For this review, take the finished solid that the model builds, in its own axes (mm). A direction names the side the tool comes from. Give positions to 0.01 mm unless a question says otherwise; leave off trailing zeros. Order: outer loops, then holes, each group sorted by start corner. A loop starts at its lowest first (then second) coordinate and runs counter-clockwise, first axis right, second up.
from build123d import *

# Parameters (mm, degrees)
SKETCH1_W           = 20
SKETCH1_H           = 90
BOSS_EXTRUDE1_DEPTH = 30
SKETCH2_W           = 40
SKETCH2_H           = 40
BOSS_EXTRUDE2_DEPTH = 20
FILLET1_R           = 10


with BuildPart() as part:
    # Sketch1 → Boss-Extrude1 (new body)
    with BuildSketch(Plane.XY):
        with Locations((-20, -45)):
            Rectangle(SKETCH1_W, SKETCH1_H)
    extrude(amount=BOSS_EXTRUDE1_DEPTH)

    # Sketch2 → Boss-Extrude2 (add)
    with BuildSketch(Plane.XY):
        with Locations((-10, -70)):
            Rectangle(SKETCH2_W, SKETCH2_H)
    extrude(amount=-BOSS_EXTRUDE2_DEPTH)

    # Fillet1
    fillet1_edges = [part.edges().sort_by_distance(p)[0] for p in [
        (10, -50, -10),
        (-20, 0, 30),
    ]]
    fillet(fillet1_edges, radius=FILLET1_R)


solid = part.part
1) We need section A-A on x = -13. Give the boundary of the cut face in (y, z), then the cut area to 3 significant figures.
Answer sheet:
outline: (-90, -20) - (-50, -20) - (-50, 0) - (0, 0) - (0, 20) arc R10 ccw to (-10, 30) - (-90, 30) - close
area: 3,480 mm2
2) Clearance check with flat-ended pins moving along their axes: pin 1 (3 mm diameter, centred on y = -59, z = 10.5, fed in from +X); pin 2 (10 mm diameter, centred on x = -4.5, y = -78.5, fed in from +Z); pin 3 (10 mm diameter, centred on x = -17, z = -10, fed in from +Y). State where each tip first meets the part, or that it passes through.
Answer sheet:
pin 1: stops at x = -10
pin 2: stops at z = 0
pin 3: stops at y = -50
3) We need section B-B on z = -3.5. Give the boundary of the cut face in (x, y), then the cut area to 3 significant figures.
Answer sheet:
outline: (-30, -90) - (10, -90) - (10, -60) arc R10 ccw to (0, -50) - (-30, -50) - close
area: 1,580 mm2
4) Tool access review of faces 1 (the face through (0, -70, 0)), 2 (the face through (-15, -90, 0)), 3 (the face through (-15, -50, -10)): name each direction out of +Z, -Z, +X, -X, +Y, -Y from which nothing blocks a thin tool from reaching the whole face with its end or side.
Answer sheet:
face 1: +Z, +X, +Y, -Y
face 2: +Z, -Z, +X, -X, -Y
face 3: -Z, +X, -X, +Y
5) We need section C-C on y = -73.5. Give the boundary of the cut face in (x, z), then the cut area to 3 significant figures.
Answer sheet:
outline: (-30, -20) - (10, -20) - (10, 0) - (-10, 0) - (-10, 30) - (-30, 30) - close
area: 1,400 mm2
6) We need section D-D on y = -54. Give the boundary of the cut face in (x, z), then the cut area to 3 significant figures.
Answer sheet:
outline: (-30, -20) - (8, -20) - (8, 0) - (-10, 0) - (-10, 30) - (-30, 30) - close
area: 1,360 mm2
7) To check wall thickness, follow line 1 (Y direction, x = -8, z = -12.5); line 2 (Z direction, x = 2.5, y = -56.5); line 3 (X direction, y = -72, z = 12.5). State the ranges of each line that lie inside material, in increasing order.
Answer sheet:
line 1: y = -90 to -50
line 2: z = -20 to 0
line 3: x = -30 to -10
